Could you check a few things on this drawing? It's one solid part, dimensions in mm from its lowest x, y, z. A direction names the side the tool comes from. Round coordinates to 2 decimals unless told otherwise and drop trailing zeros. Loops run counter-clockwise (first coordinate to the right, second up) from the corner with the lowest first, then second, coordinate; pieces in that order, holes last. Notation, with made-up numbers: M 58,1.5 L 78,1.5 A14 cw 78,19.5 Z; hole C 35,14.25 d4. An arc over 180 degrees is marked long. Write item = value, one per line. Start each with the question number.
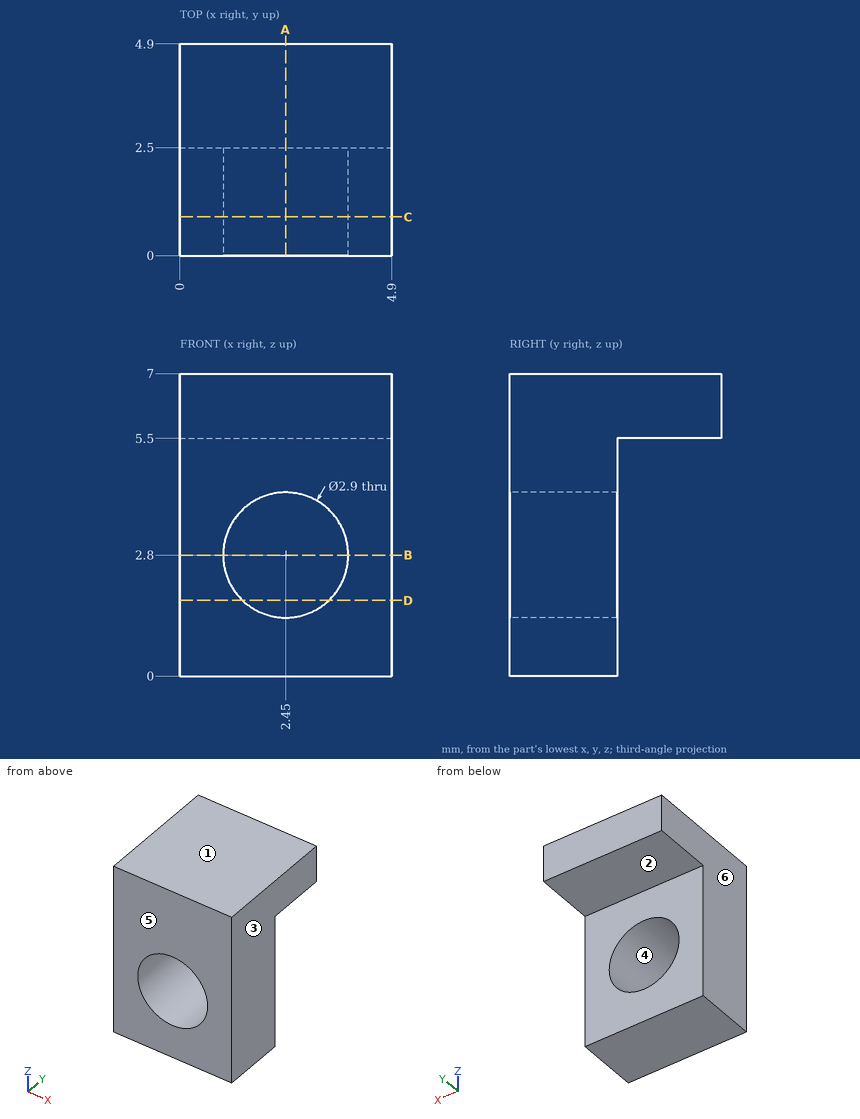
Item 1: For the marked faces 1 and 2, which set-ups out of +Z, -Z, +X, -X, +Y, -Y let a thin tool reach every point of the face, with its end or its side?
Item 2: I want a section at B-B, the plane z = 2.8. List the corners of the cut face in (x, y) for me.
Item 3: We'd pull the mould along X, two halves only. Please class the marked faces 3, 4, 5 and 6: released by +X, released by -X, zero draft, split by the parting line, or undercut.
Item 4: I want a section at C-C, the plane y = 0.9. List the corners of the cut face in (x, z) for me, then the cut area to 3 significant figures.
Item 5: I want a section at D-D, the plane z = 1.75. List the corners of the cut face in (x, y) for me, then the cut area to 3 significant figures.
Item 6: Please list where these lines run through material, in increasing order: line 1 (Z direction, x = 2.45, y = 1.1); line 2 (Y direction, x = 3.95, z = 3.75); line 3 (X direction, y = 1.5, z = 3.25). Write a range as [from, to].
Item 7: I want a section at A-A, the plane x = 2.45. List the corners of the cut face in (y, z) for me.
Worked out:
q1.face_1 = +Z, +X, -X, +Y, -Y
q1.face_2 = -Z, +X, -X, +Y
q2.outline = M 0,0 L 1,0 L 1,2.5 L 0,2.5 Z; M 3.9,0 L 4.9,0 L 4.9,2.5 L 3.9,2.5 Z
q3.face_3 = released by +X
q3.face_4 = undercut
q3.face_5 = zero draft
q3.face_6 = released by -X
q4.outline = M 0,0 L 4.9,0 L 4.9,7 L 0,7 Z; hole C 2.45,2.8 d2.9
q4.area = 27.7 mm2
q5.outline = M 0,0 L 1.45,0 L 1.45,2.5 L 0,2.5 Z; M 3.45,0 L 4.9,0 L 4.9,2.5 L 3.45,2.5 Z
q5.area = 7.25 mm2
q6.line_1 = [0, 1.35], [4.25, 7]
q6.line_2 = [0, 2.5]
q6.line_3 = [0, 1.07], [3.83, 4.9]
q7.outline = M 0,0 L 2.5,0 L 2.5,1.35 L 0,1.35 Z; M 0,4.25 L 2.5,4.25 L 2.5,5.5 L 4.9,5.5 L 4.9,7 L 0,7 Z
